Geometry: see drawing. Coordinates: mm, zero at the bounding-box minimum. A direction names the side the tool comes from. Round coordinates to 2 decimals unless told otherwise and drop trailing zeros. Write each loop counter-clockwise with the first axis right and the second up, starting at its lowest first coordinate (ties: lowest second). Pieces come first, ordered by that corner, then holes.
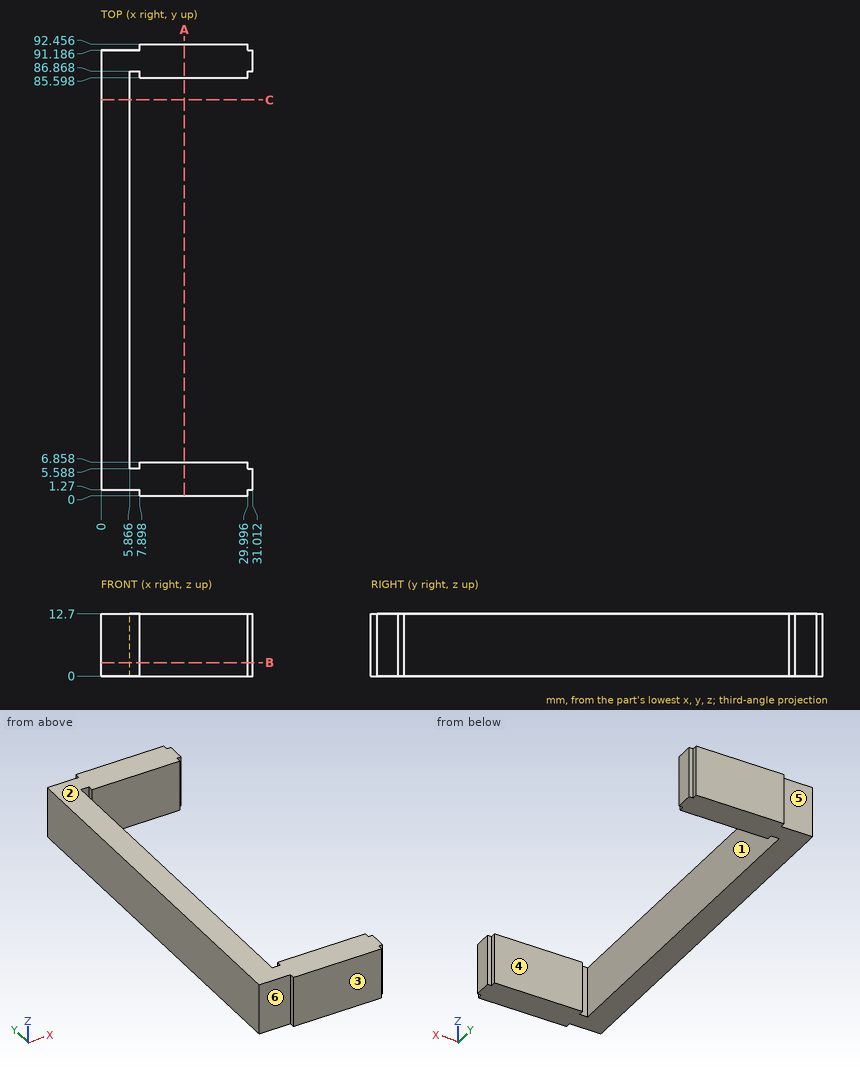
1) Section query C-C on y = 81. Return the cut outline in (x, z).
Taken from the geometry:
outline: (0, 0) - (5.87, 0) - (5.87, 12.7) - (0, 12.7) - close
2) Reachability of the marked faces 4, 5 and 6 from +Z, -Z, +X, -X, +Y, -Y: full face, straight path, thin tool, end or side. Return the list, or none.
Taken from the geometry:
face 4: +Z, -Z, +X
face 5: +Z, -Z, -X, +Y
face 6: +Z, -Z, -X, -Y
3) Section query A-A on x = 17. Return the cut outline in (y, z).
Taken from the geometry:
outline: (0, 0) - (6.86, 0) - (6.86, 12.7) - (0, 12.7) - close; (85.6, 0) - (92.46, 0) - (92.46, 12.7) - (85.6, 12.7) - close
4) Contact query for flat-ended pins moving along their axis: P1, Ø1, axis at x = 6.5, z = 8.5, coming from the +Y side; P2, Ø0.5, axis at x = 30.5, z = 7, coming from the -Y side; P3, Ø1, axis at y = 0.5, z = 7.5, coming from the -X side. Output: stop coordinate, or through.
Taken from the geometry:
P1: stops at y = 91.19
P2: stops at y = 1.27
P3: stops at x = 7.9
5) Material intervals for line 1 (Y direction, x = 16.5, z = 2.25); line 2 (X direction, y = 30.5, z = 1.75); line 3 (Y direction, x = 3.5, z = 2), sorted ascending.
Taken from the geometry:
line 1: y = 0 to 6.86, 85.6 to 92.46
line 2: x = 0 to 5.87
line 3: y = 1.27 to 91.19
6) Section query B-B on z = 2.75. Return the cut outline in (x, y), then the cut area to 3 significant figures.
Taken from the geometry:
outline: (0, 1.27) - (7.9, 1.27) - (7.9, 0) - (30, 0) - (30, 1.27) - (31.01, 1.27) - (31.01, 5.59) - (30, 5.59) - (30, 6.86) - (7.9, 6.86) - (7.9, 5.59) - (5.87, 5.59) - (5.87, 86.87) - (7.9, 86.87) - (7.9, 85.6) - (30, 85.6) - (30, 86.87) - (31.01, 86.87) - (31.01, 91.19) - (30, 91.19) - (30, 92.46) - (7.9, 92.46) - (7.9, 91.19) - (0, 91.19) - close
area: 857 mm2
7) Pull-direction query (Y, two-part tool) for the marked faces 1, 2 and 3; classes: released by +Y, released by -Y, zero draft, split by the parting line, or undercut.
Taken from the geometry:
face 1: undercut
face 2: zero draft
face 3: released by -Y
